from build123d import *

# Parameters (mm, degrees)
CROQUIS1_W              = 38
CROQUIS1_H              = 38
CROQUIS1_W_2            = 28
CROQUIS1_H_2            = 28
SALIENTE_EXTRUIR1_DEPTH = 1020
CORTAR_EXTRUIR1_REACH   = 1022.884
CROQUIS2_R              = 2.87


with BuildPart() as part:
    # Croquis1 → Saliente-Extruir1 (new body)
    with BuildSketch(Plane.XY):
        Rectangle(CROQUIS1_W, CROQUIS1_H)
        Rectangle(CROQUIS1_W_2, CROQUIS1_H_2, mode=Mode.SUBTRACT)
    extrude(amount=SALIENTE_EXTRUIR1_DEPTH)

    # Cortar-Extruir1: up to this face of the body (flat: up to its plane)
    cortar_extruir1_end = Plane(part.part.faces().sort_by_distance((0, -19, 510))[0])
    # Croquis2 → Cortar-Extruir1 (cut, up to the picked face)
    with BuildSketch(Plane(origin=(0, 19, 0), x_dir=(1, 0, 0), z_dir=(0, 1, 0)), mode=Mode.PRIVATE) as cortar_extruir1_sk1:
        with Locations(Location((0, -30.72, 0), (0, 0, 270))):
            Circle(CROQUIS2_R)
    cortar_extruir1_tool1 = split(extrude(cortar_extruir1_sk1.sketch, amount=-CORTAR_EXTRUIR1_REACH, mode=Mode.PRIVATE), bisect_by=cortar_extruir1_end, keep=Keep.BOTH, mode=Mode.PRIVATE)
    # Croquis2 → Cortar-Extruir1 (cut, up to the picked face)
    with BuildSketch(Plane(origin=(0, 19, 0), x_dir=(1, 0, 0), z_dir=(0, 1, 0)), mode=Mode.PRIVATE) as cortar_extruir1_sk2:
        with Locations(Location((0, -90.63, 0), (0, 0, 270))):
            Circle(CROQUIS2_R)
    cortar_extruir1_tool2 = split(extrude(cortar_extruir1_sk2.sketch, amount=-CORTAR_EXTRUIR1_REACH, mode=Mode.PRIVATE), bisect_by=cortar_extruir1_end, keep=Keep.BOTH, mode=Mode.PRIVATE)
    # Croquis2 → Cortar-Extruir1 (cut, up to the picked face)
    with BuildSketch(Plane(origin=(0, 19, 0), x_dir=(1, 0, 0), z_dir=(0, 1, 0)), mode=Mode.PRIVATE) as cortar_extruir1_sk3:
        with Locations(Location((0, -150.54, 0), (0, 0, 270))):
            Circle(CROQUIS2_R)
    cortar_extruir1_tool3 = split(extrude(cortar_extruir1_sk3.sketch, amount=-CORTAR_EXTRUIR1_REACH, mode=Mode.PRIVATE), bisect_by=cortar_extruir1_end, keep=Keep.BOTH, mode=Mode.PRIVATE)
    # Croquis2 → Cortar-Extruir1 (cut, up to the picked face)
    with BuildSketch(Plane(origin=(0, 19, 0), x_dir=(1, 0, 0), z_dir=(0, 1, 0)), mode=Mode.PRIVATE) as cortar_extruir1_sk4:
        with Locations(Location((0, -210.45, 0), (0, 0, 270))):
            Circle(CROQUIS2_R)
    cortar_extruir1_tool4 = split(extrude(cortar_extruir1_sk4.sketch, amount=-CORTAR_EXTRUIR1_REACH, mode=Mode.PRIVATE), bisect_by=cortar_extruir1_end, keep=Keep.BOTH, mode=Mode.PRIVATE)
    # Croquis2 → Cortar-Extruir1 (cut, up to the picked face)
    with BuildSketch(Plane(origin=(0, 19, 0), x_dir=(1, 0, 0), z_dir=(0, 1, 0)), mode=Mode.PRIVATE) as cortar_extruir1_sk5:
        with Locations(Location((0, -270.36, 0), (0, 0, 270))):
            Circle(CROQUIS2_R)
    cortar_extruir1_tool5 = split(extrude(cortar_extruir1_sk5.sketch, amount=-CORTAR_EXTRUIR1_REACH, mode=Mode.PRIVATE), bisect_by=cortar_extruir1_end, keep=Keep.BOTH, mode=Mode.PRIVATE)
    # Croquis2 → Cortar-Extruir1 (cut, up to the picked face)
    with BuildSketch(Plane(origin=(0, 19, 0), x_dir=(1, 0, 0), z_dir=(0, 1, 0)), mode=Mode.PRIVATE) as cortar_extruir1_sk6:
        with Locations(Location((0, -330.27, 0), (0, 0, 270))):
            Circle(CROQUIS2_R)
    cortar_extruir1_tool6 = split(extrude(cortar_extruir1_sk6.sketch, amount=-CORTAR_EXTRUIR1_REACH, mode=Mode.PRIVATE), bisect_by=cortar_extruir1_end, keep=Keep.BOTH, mode=Mode.PRIVATE)
    # Croquis2 → Cortar-Extruir1 (cut, up to the picked face)
    with BuildSketch(Plane(origin=(0, 19, 0), x_dir=(1, 0, 0), z_dir=(0, 1, 0)), mode=Mode.PRIVATE) as cortar_extruir1_sk7:
        with Locations(Location((0, -390.18, 0), (0, 0, 270))):
            Circle(CROQUIS2_R)
    cortar_extruir1_tool7 = split(extrude(cortar_extruir1_sk7.sketch, amount=-CORTAR_EXTRUIR1_REACH, mode=Mode.PRIVATE), bisect_by=cortar_extruir1_end, keep=Keep.BOTH, mode=Mode.PRIVATE)
    # Croquis2 → Cortar-Extruir1 (cut, up to the picked face)
    with BuildSketch(Plane(origin=(0, 19, 0), x_dir=(1, 0, 0), z_dir=(0, 1, 0)), mode=Mode.PRIVATE) as cortar_extruir1_sk8:
        with Locations(Location((0, -450.09, 0), (0, 0, 270))):
            Circle(CROQUIS2_R)
    cortar_extruir1_tool8 = split(extrude(cortar_extruir1_sk8.sketch, amount=-CORTAR_EXTRUIR1_REACH, mode=Mode.PRIVATE), bisect_by=cortar_extruir1_end, keep=Keep.BOTH, mode=Mode.PRIVATE)
    # Croquis2 → Cortar-Extruir1 (cut, up to the picked face)
    with BuildSketch(Plane(origin=(0, 19, 0), x_dir=(1, 0, 0), z_dir=(0, 1, 0)), mode=Mode.PRIVATE) as cortar_extruir1_sk9:
        with Locations(Location((0, -510, 0), (0, 0, 270))):
            Circle(CROQUIS2_R)
    cortar_extruir1_tool9 = split(extrude(cortar_extruir1_sk9.sketch, amount=-CORTAR_EXTRUIR1_REACH, mode=Mode.PRIVATE), bisect_by=cortar_extruir1_end, keep=Keep.BOTH, mode=Mode.PRIVATE)
    # Croquis2 → Cortar-Extruir1 (cut, up to the picked face)
    with BuildSketch(Plane(origin=(0, 19, 0), x_dir=(1, 0, 0), z_dir=(0, 1, 0)), mode=Mode.PRIVATE) as cortar_extruir1_sk10:
        with Locations(Location((0, -569.91, 0), (0, 0, 270))):
            Circle(CROQUIS2_R)
    cortar_extruir1_tool10 = split(extrude(cortar_extruir1_sk10.sketch, amount=-CORTAR_EXTRUIR1_REACH, mode=Mode.PRIVATE), bisect_by=cortar_extruir1_end, keep=Keep.BOTH, mode=Mode.PRIVATE)
    # Croquis2 → Cortar-Extruir1 (cut, up to the picked face)
    with BuildSketch(Plane(origin=(0, 19, 0), x_dir=(1, 0, 0), z_dir=(0, 1, 0)), mode=Mode.PRIVATE) as cortar_extruir1_sk11:
        with Locations(Location((0, -629.82, 0), (0, 0, 270))):
            Circle(CROQUIS2_R)
    cortar_extruir1_tool11 = split(extrude(cortar_extruir1_sk11.sketch, amount=-CORTAR_EXTRUIR1_REACH, mode=Mode.PRIVATE), bisect_by=cortar_extruir1_end, keep=Keep.BOTH, mode=Mode.PRIVATE)
    # Croquis2 → Cortar-Extruir1 (cut, up to the picked face)
    with BuildSketch(Plane(origin=(0, 19, 0), x_dir=(1, 0, 0), z_dir=(0, 1, 0)), mode=Mode.PRIVATE) as cortar_extruir1_sk12:
        with Locations(Location((0, -689.73, 0), (0, 0, 270))):
            Circle(CROQUIS2_R)
    cortar_extruir1_tool12 = split(extrude(cortar_extruir1_sk12.sketch, amount=-CORTAR_EXTRUIR1_REACH, mode=Mode.PRIVATE), bisect_by=cortar_extruir1_end, keep=Keep.BOTH, mode=Mode.PRIVATE)
    # Croquis2 → Cortar-Extruir1 (cut, up to the picked face)
    with BuildSketch(Plane(origin=(0, 19, 0), x_dir=(1, 0, 0), z_dir=(0, 1, 0)), mode=Mode.PRIVATE) as cortar_extruir1_sk13:
        with Locations(Location((0, -749.64, 0), (0, 0, 270))):
            Circle(CROQUIS2_R)
    cortar_extruir1_tool13 = split(extrude(cortar_extruir1_sk13.sketch, amount=-CORTAR_EXTRUIR1_REACH, mode=Mode.PRIVATE), bisect_by=cortar_extruir1_end, keep=Keep.BOTH, mode=Mode.PRIVATE)
    # Croquis2 → Cortar-Extruir1 (cut, up to the picked face)
    with BuildSketch(Plane(origin=(0, 19, 0), x_dir=(1, 0, 0), z_dir=(0, 1, 0)), mode=Mode.PRIVATE) as cortar_extruir1_sk14:
        with Locations(Location((0, -809.55, 0), (0, 0, 270))):
            Circle(CROQUIS2_R)
    cortar_extruir1_tool14 = split(extrude(cortar_extruir1_sk14.sketch, amount=-CORTAR_EXTRUIR1_REACH, mode=Mode.PRIVATE), bisect_by=cortar_extruir1_end, keep=Keep.BOTH, mode=Mode.PRIVATE)
    # Croquis2 → Cortar-Extruir1 (cut, up to the picked face)
    with BuildSketch(Plane(origin=(0, 19, 0), x_dir=(1, 0, 0), z_dir=(0, 1, 0)), mode=Mode.PRIVATE) as cortar_extruir1_sk15:
        with Locations(Location((0, -869.46, 0), (0, 0, 270))):
            Circle(CROQUIS2_R)
    cortar_extruir1_tool15 = split(extrude(cortar_extruir1_sk15.sketch, amount=-CORTAR_EXTRUIR1_REACH, mode=Mode.PRIVATE), bisect_by=cortar_extruir1_end, keep=Keep.BOTH, mode=Mode.PRIVATE)
    # Croquis2 → Cortar-Extruir1 (cut, up to the picked face)
    with BuildSketch(Plane(origin=(0, 19, 0), x_dir=(1, 0, 0), z_dir=(0, 1, 0)), mode=Mode.PRIVATE) as cortar_extruir1_sk16:
        with Locations(Location((0, -929.37, 0), (0, 0, 270))):
            Circle(CROQUIS2_R)
    cortar_extruir1_tool16 = split(extrude(cortar_extruir1_sk16.sketch, amount=-CORTAR_EXTRUIR1_REACH, mode=Mode.PRIVATE), bisect_by=cortar_extruir1_end, keep=Keep.BOTH, mode=Mode.PRIVATE)
    # Croquis2 → Cortar-Extruir1 (cut, up to the picked face)
    with BuildSketch(Plane(origin=(0, 19, 0), x_dir=(1, 0, 0), z_dir=(0, 1, 0)), mode=Mode.PRIVATE) as cortar_extruir1_sk17:
        with Locations(Location((0, -989.28, 0), (0, 0, 270))):
            Circle(CROQUIS2_R)
    cortar_extruir1_tool17 = split(extrude(cortar_extruir1_sk17.sketch, amount=-CORTAR_EXTRUIR1_REACH, mode=Mode.PRIVATE), bisect_by=cortar_extruir1_end, keep=Keep.BOTH, mode=Mode.PRIVATE)
    add(cortar_extruir1_tool1.solids().sort_by(Axis((0, 19, 30.72), (0, -1, 0)))[0], mode=Mode.SUBTRACT)
    add(cortar_extruir1_tool2.solids().sort_by(Axis((0, 19, 90.63), (0, -1, 0)))[0], mode=Mode.SUBTRACT)
    add(cortar_extruir1_tool3.solids().sort_by(Axis((0, 19, 150.54), (0, -1, 0)))[0], mode=Mode.SUBTRACT)
    add(cortar_extruir1_tool4.solids().sort_by(Axis((0, 19, 210.45), (0, -1, 0)))[0], mode=Mode.SUBTRACT)
    add(cortar_extruir1_tool5.solids().sort_by(Axis((0, 19, 270.36), (0, -1, 0)))[0], mode=Mode.SUBTRACT)
    add(cortar_extruir1_tool6.solids().sort_by(Axis((0, 19, 330.27), (0, -1, 0)))[0], mode=Mode.SUBTRACT)
    add(cortar_extruir1_tool7.solids().sort_by(Axis((0, 19, 390.18), (0, -1, 0)))[0], mode=Mode.SUBTRACT)
    add(cortar_extruir1_tool8.solids().sort_by(Axis((0, 19, 450.09), (0, -1, 0)))[0], mode=Mode.SUBTRACT)
    add(cortar_extruir1_tool9.solids().sort_by(Axis((0, 19, 510), (0, -1, 0)))[0], mode=Mode.SUBTRACT)
    add(cortar_extruir1_tool10.solids().sort_by(Axis((0, 19, 569.91), (0, -1, 0)))[0], mode=Mode.SUBTRACT)
    add(cortar_extruir1_tool11.solids().sort_by(Axis((0, 19, 629.82), (0, -1, 0)))[0], mode=Mode.SUBTRACT)
    add(cortar_extruir1_tool12.solids().sort_by(Axis((0, 19, 689.73), (0, -1, 0)))[0], mode=Mode.SUBTRACT)
    add(cortar_extruir1_tool13.solids().sort_by(Axis((0, 19, 749.64), (0, -1, 0)))[0], mode=Mode.SUBTRACT)
    add(cortar_extruir1_tool14.solids().sort_by(Axis((0, 19, 809.55), (0, -1, 0)))[0], mode=Mode.SUBTRACT)
    add(cortar_extruir1_tool15.solids().sort_by(Axis((0, 19, 869.46), (0, -1, 0)))[0], mode=Mode.SUBTRACT)
    add(cortar_extruir1_tool16.solids().sort_by(Axis((0, 19, 929.37), (0, -1, 0)))[0], mode=Mode.SUBTRACT)
    add(cortar_extruir1_tool17.solids().sort_by(Axis((0, 19, 989.28), (0, -1, 0)))[0], mode=Mode.SUBTRACT)


solid = part.part
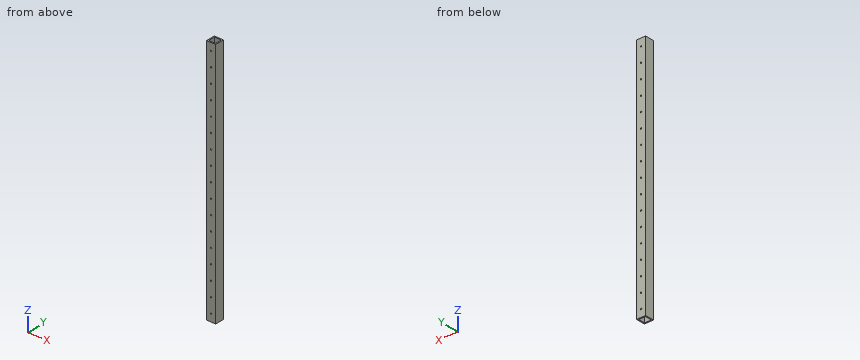
Build history of the part. All positions in model axes, mm. Round coordinates to 2 decimals unless told otherwise and drop trailing zeros. Write each loop counter-clockwise with the first axis right and the second up, starting at its lowest first coordinate (ties: lowest second). Pieces come first, ordered by that corner, then holes. Notation, with made-up numbers: M -21,11 L -12,11 A28 cw -12,30 Z; hole C 53,-1 d8. An arc over 180 degrees is marked long. Answer in a Markdown table with one row per item.
1. Flat gauge pin, fed straight in: P1, Ø6.5, axis at x = 0, z = 510, coming from the +Y side. Where does the tip first touch, or does it go through?
Geometry check:
| item | result |
|---|---|
| P1 | y = 19 |
2. Saw through at A-A (z = 582.5). List the corners of the cut face in (x, y), and give its area (3 significant figures).
Geometry check:
| item | result |
|---|---|
| outline | M -19,-19 L 19,-19 L 19,19 L -19,19 Z; hole M -14,-14 L 14,-14 L 14,14 L -14,14 Z |
| area | 660 mm2 |
3. Probe L1, parallel to X at y = -10, z = 48; L2, parallel to X at y = -17.1, z = 450.09. List the from-to ranges inside material, lowest first. Write a range as [from, to].
Geometry check:
| item | result |
|---|---|
| L1 | [-19, -14], [14, 19] |
| L2 | [-19, -2.87], [2.87, 19] |
